For this review, take the finished solid that the model builds, in its own axes (mm). A direction names the side the tool comes from. Round coordinates to 2 decimals unless told otherwise and drop trailing zeros. Order: outer loops, then holes, each group sorted by start corner. A loop starts at its lowest first (then second) coordinate and runs counter-clockwise, first axis right, second up. Notation, with made-up numbers: (30, 1) - (72, 1) arc R29 cw to (72, 23) - close; hole circle Ø3 at (27, 62.25). An arc over 180 degrees is marked (long way). Write each question's results on one line, items separated by ' | '. Start each with the question number.
(1) For L1, parallel to Z at x = 36, y = 31; L2, parallel to Z at x = 6.5, y = 29.5; L3, parallel to Z at x = 15, y = 20, list the stretches that pass through material, from the lowest coordinate up. Write a range as from..to.
(2) Insertion check: pin 1 Ø24 at (x, z) = (-5.5, 71) entering from +Y; pin 2 Ø1.5 at (y, z) = (17.5, 56.5) entering from +X; pin 3 Ø1 at (x, y) = (49.5, 16) entering from +Z. Each pin has a flat end and moves straight along its axis. Give the tip position at first contact, or say it passes through.
(3) Draft analysis for pull direction Y (two halves, no side actions). For faces 4 (the flat face through (22, 39, 21.082)), 5 (the cylindrical face through (0.318, 17.739, 64.482)), 6 (the flat face through (22, 0, 65)), 7 (the flat face through (37.85, 33.75, 10.39)), state which applies: pulls with the +Y half, pulls with the -Y half, needs draft (parallel to the pull), parting line crosses it, or undercut.
(4) Take a section at C-C, the plane x = 17.5. Give the boundary of the cut face in (y, z), plus the area to 3 significant figures.
(5) Take a section at A-A, the plane y = 36.5. Give the boundary of the cut face in (x, z).
(6) Take a section at D-D, the plane x = 29.5. Give the boundary of the cut face in (y, z), plus the area to 3 significant figures.
(7) For faces 1 (the flat face through (30.14, 28.74, 77.36)), 2 (the flat face through (-9, 56.688, 77)), 3 (the flat face through (11, 27, 0)), list the 3-axis set-ups (+Z, -Z, +X, -X, +Y, -Y) from which the entire face can be reached by the end or side of a thin tool; tool diameter is ignored.
(8) Take a section at B-B, the plane z = 53. Give the boundary of the cut face in (x, y).
```python
from build123d import *

# Parameters (mm, degrees)
F1_DEPTH = 132.08
F3_DEPTH = 110.998
F4_R     = 10.950567
F5_DEPTH = 77.47


with BuildPart() as f1:
    # F0 (on Top) → F1 (new body)
    with BuildSketch(Plane.XY):
        Polygon((-24.245454, 68.464547), (-24.245454, 0), (68.81091, 0), (6.003636, 68.464547), align=None)
    extrude(amount=F1_DEPTH)

    # F2 (on face) → F3 (cut)
    with BuildSketch(Plane.XY.offset(132.08)):
        Polygon((-24.245454, 68.464547), (-24.245454, 56.688186), (6.003636, 56.688186), (54.956365, 0), (68.81091, 0), (6.003636, 68.464547), align=None)
    extrude(amount=-F3_DEPTH, mode=Mode.SUBTRACT)

    # F4 (on face) → F5 (cut)
    with BuildSketch(Plane(origin=(-24.245454, 0, 0), x_dir=(0, -1, 0), z_dir=(-1, 0, 0))):
        with Locations((-28.183466, 61.193019)):
            Circle(F4_R)
    extrude(amount=-F5_DEPTH, mode=Mode.SUBTRACT)


solid = f1.part
```
Results below:
1) L1: z = 0..21.08 | L2: z = 0..50.32, 72.06..132.08 | L3: z = 0..53.92, 68.47..132.08
2) pin 1: stops at y = 56.69 | pin 2: stops at x = 40.49 | pin 3: stops at z = 21.08
3) face 4: needs draft | face 5: undercut | face 6: pulls with the -Y half | face 7: pulls with the +Y half
4) outline: (0, 0) - (55.93, 0) - (55.93, 21.08) - (43.38, 21.08) - (43.38, 132.08) - (0, 132.08) - close; hole circle Ø21.9 at (28.18, 61.19) | area: 5,620 mm^2
5) outline: (-24.25, 0) - (35.33, 0) - (35.33, 21.08) - (23.44, 21.08) - (23.44, 54.07) - (-24.25, 54.07) - close; (-24.25, 68.32) - (23.44, 68.32) - (23.44, 132.08) - (-24.25, 132.08) - close
6) outline: (0, 0) - (42.85, 0) - (42.85, 21.08) - (29.48, 21.08) - (29.48, 50.32) arc R10.95 cw (long way) to (29.48, 72.07) - (29.48, 132.08) - (0, 132.08) - close | area: 3,960 mm^2
7) face 1: +Z, +X, +Y | face 2: +Z, +X, -X, +Y | face 3: -Z, +X, -X, +Y, -Y
8) outline: (-24.25, 0) - (54.96, 0) - (36.89, 20.92) - (-24.25, 20.92) - close; (-24.25, 35.45) - (24.34, 35.45) - (6, 56.69) - (-24.25, 56.69) - close
